Build history of the part. All positions in model axes, mm. Face numbers are marked on the shaded views. A direction names the side the tool comes from. Round coordinates to 2 decimals unless told otherwise and drop trailing zeros. Write each loop counter-clockwise with the first axis right and the second up, starting at its lowest first coordinate (ties: lowest second). Pieces come first, ordered by that corner, then holes. Notation, with made-up numbers: (63.25, 39.5) - (113.25, 39.5) arc R24 cw to (113.25, 78.5) - close; hole circle Ø9 at (-18.5, -12.75). An arc over 180 degrees is marked (long way). Write each question's results on one line, items separated by ' | '.
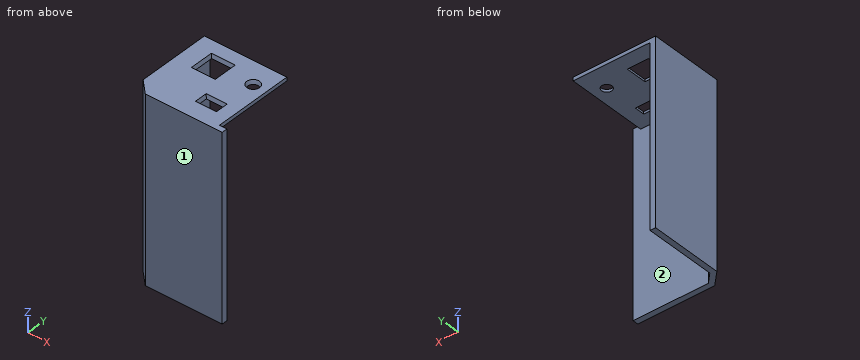
from build123d import *

# Parameters (mm, degrees)
BOSS_EXTRUDE1_DEPTH          = 100
BOSS_EXTRUDE2_DEPTH          = 2
CUT_EXTRUDE2_REACH           = 120.237
SKETCH4_R                    = 2.75
CUT_EXTRUDE3_REACH           = 120.237
SKETCH5_W                    = 9
SKETCH5_H                    = 4
CUT_EXTRUDE4_REACH           = 120.237
SKETCH6_W                    = 10
SKETCH6_H                    = 10
SKETCH7_R                    = 3.5
CUT_EXTRUDE6_DEPTH           = 2
CUT_EXTRUDE6_DRAFT           = -20
SKETCH7_W                    = 11.447026043
SKETCH7_H                    = 7
CUT_EXTRUDE6_PROFILE_2_DEPTH = 2
CUT_EXTRUDE6_PROFILE_2_DRAFT = -20
SKETCH7_W_2                  = 13
SKETCH7_H_2                  = 13
CUT_EXTRUDE6_PROFILE_3_DEPTH = 2
CUT_EXTRUDE6_PROFILE_3_DRAFT = -20


with BuildPart() as part:
    # Sketch2 → Boss-Extrude1 (new body)
    with BuildSketch(Plane.XY):
        Polygon((-7.071067812, 47.073759399), (-4.071067812, 47.073759399), (-4.071067812, 8.071067812), (1, 3), (42, 3), (42, 0), (0, 0), (-7.071067812, 7.071067812), align=None)
    extrude(amount=BOSS_EXTRUDE1_DEPTH)

    # Sketch3 → Boss-Extrude2 (add)
    with BuildSketch(Plane.XY.offset(100)):
        Polygon((-4.071067812, 47.073759399), (37.928932188, 47.073759399), (37.928932188, 3), (1, 3), (-4.071067812, 8.071067812), align=None)
    extrude(amount=-BOSS_EXTRUDE2_DEPTH)

    # Sketch4 → Cut-Extrude2 (cut, up to next)
    with BuildSketch(Plane.XY.offset(100), mode=Mode.PRIVATE) as cut_extrude2_sk1:
        with Locations((30.428932188, 34.073759399)):
            Circle(SKETCH4_R)
    cut_extrude2_tool1 = extrude(cut_extrude2_sk1.sketch, amount=-CUT_EXTRUDE2_REACH, mode=Mode.PRIVATE) & part.part
    add(cut_extrude2_tool1.solids().sort_by_distance((30.428932, 34.073759, 100))[0], mode=Mode.SUBTRACT)

    # Sketch5 → Cut-Extrude3 (cut, up to next)
    with BuildSketch(Plane.XY.offset(100), mode=Mode.PRIVATE) as cut_extrude3_sk1:
        with Locations((25.428932188, 13)):
            Rectangle(SKETCH5_W, SKETCH5_H)
    cut_extrude3_tool1 = extrude(cut_extrude3_sk1.sketch, amount=-CUT_EXTRUDE3_REACH, mode=Mode.PRIVATE) & part.part
    add(cut_extrude3_tool1.solids().sort_by_distance((25.428932, 13, 100))[0], mode=Mode.SUBTRACT)

    # Sketch6 → Cut-Extrude4 (cut, up to next)
    with BuildSketch(Plane.XY.offset(100), mode=Mode.PRIVATE) as cut_extrude4_sk1:
        with Locations((9.428932188, 33.144002223)):
            Rectangle(SKETCH6_W, SKETCH6_H)
    cut_extrude4_tool1 = extrude(cut_extrude4_sk1.sketch, amount=-CUT_EXTRUDE4_REACH, mode=Mode.PRIVATE) & part.part
    add(cut_extrude4_tool1.solids().sort_by_distance((9.428932, 33.144002, 100))[0], mode=Mode.SUBTRACT)


with BuildPart() as cut_extrude6_tool:
    # Sketch7 → Cut-Extrude6 (with draft: the straight prism first)
    with BuildSketch(Plane.XY.offset(100)):
        with Locations((30.428932188, 34.073759399)):
            Circle(SKETCH7_R)
    extrude(amount=-CUT_EXTRUDE6_DEPTH)
    # Cut-Extrude6: the draft: its side faces are tilted about the plane it starts from
    cut_extrude6_sides = [cut_extrude6_tool.faces().sort_by_distance(p)[0] for p in [
        (26.928932188, 34.073759399, 99),
    ]]
    draft(cut_extrude6_sides, Plane.XY.offset(100), CUT_EXTRUDE6_DRAFT)


with BuildPart() as part_1:
    add(part.part)

    # Cut-Extrude6: cut by cut_extrude6_tool
    add(cut_extrude6_tool.part, mode=Mode.SUBTRACT)


with BuildPart() as cut_extrude6_profile_2_tool:
    # Sketch7 → Cut-Extrude6 profile 2 (with draft: the straight prism first)
    with BuildSketch(Plane.XY.offset(100)):
        with Locations((25.15244521, 13)):
            Rectangle(SKETCH7_W, SKETCH7_H)
    extrude(amount=-CUT_EXTRUDE6_PROFILE_2_DEPTH)
    # Cut-Extrude6 profile 2: the draft: its side faces are tilted about the plane it starts from
    cut_extrude6_profile_2_sides = [cut_extrude6_profile_2_tool.faces().sort_by_distance(p)[0] for p in [
        (19.428932188, 13, 99),
        (25.15244521, 9.5, 99),
        (30.875958231, 13, 99),
        (25.15244521, 16.5, 99),
    ]]
    draft(cut_extrude6_profile_2_sides, Plane.XY.offset(100), CUT_EXTRUDE6_PROFILE_2_DRAFT)


with BuildPart() as part_2:
    add(part_1.part)

    # Cut-Extrude6 profile 2: cut by cut_extrude6_profile_2_tool
    add(cut_extrude6_profile_2_tool.part, mode=Mode.SUBTRACT)


with BuildPart() as cut_extrude6_profile_3_tool:
    # Sketch7 → Cut-Extrude6 profile 3 (with draft: the straight prism first)
    with BuildSketch(Plane.XY.offset(100)):
        with Locations((9.428932188, 33.144002223)):
            Rectangle(SKETCH7_W_2, SKETCH7_H_2)
    extrude(amount=-CUT_EXTRUDE6_PROFILE_3_DEPTH)
    # Cut-Extrude6 profile 3: the draft: its side faces are tilted about the plane it starts from
    cut_extrude6_profile_3_sides = [cut_extrude6_profile_3_tool.faces().sort_by_distance(p)[0] for p in [
        (2.928932188, 33.144002223, 99),
        (9.428932188, 26.644002223, 99),
        (15.928932188, 33.144002223, 99),
        (9.428932188, 39.644002223, 99),
    ]]
    draft(cut_extrude6_profile_3_sides, Plane.XY.offset(100), CUT_EXTRUDE6_PROFILE_3_DRAFT)


with BuildPart() as part_3:
    add(part_2.part)

    # Cut-Extrude6 profile 3: cut by cut_extrude6_profile_3_tool
    add(cut_extrude6_profile_3_tool.part, mode=Mode.SUBTRACT)


solid = part_3.part
(1) Drill centre lines: probe 1 along Z at (x, y) = (1, 36); probe 2 along X at (y, z) = (34, 77); probe 3 along Y at (x, z) = (20.5, 65). Where is each one in solid material? Low to high. Write a range as [from, to].
Worked answers:
probe 1: z = [98, 100] | probe 2: x = [-7.07, -4.07] | probe 3: y = [0, 3]
(2) Flat gauge pins, fed straight in: pin 1 Ø6 at (x, y) = (36, 21) entering from -Z; pin 2 Ø8 at (y, z) = (24.5, 51) entering from +X; pin 3 Ø2 at (y, z) = (21, 99) entering from +X. Where does each tip first touch, or does it go through?
Worked answers:
pin 1: stops at z = 98 | pin 2: stops at x = -4.07 | pin 3: stops at x = 37.93
(3) Slice it at D-D, the plane z = 46. Write the cut outline in (x, y).
Worked answers:
outline: (-7.07, 7.07) - (0, 0) - (42, 0) - (42, 3) - (1, 3) - (-4.07, 8.07) - (-4.07, 47.07) - (-7.07, 47.07) - close
(4) Slice it at B-B, the plane x = 25. Write the cut outline in (y, z), and give its area (3 significant figures).
Worked answers:
outline: (0, 0) - (3, 0) - (3, 98) - (10.23, 98) - (9.5, 100) - (0, 100) - close; (15.77, 98) - (47.07, 98) - (47.07, 100) - (16.5, 100) - close | area: 376 mm2
(5) Tool access for the marked faces 1 and 2: list every direction of +Z, -Z, +X, -X, +Y, -Y with a clear straight run to the whole face (end or side of a thin tool).
Worked answers:
face 1: +Z, -Z, +X, -X, -Y | face 2: -Z, +X, +Y
(6) Slice it at C-C, the plane y = 24.5. Write the cut outline in (x, z).
Worked answers:
outline: (-7.07, 0) - (-4.07, 0) - (-4.07, 98) - (37.93, 98) - (37.93, 100) - (-7.07, 100) - close
(7) Slice it at A-A, the plane y = 12.5. Write the cut outline in (x, z), and give its area (3 significant figures).
Worked answers:
outline: (-7.07, 0) - (-4.07, 0) - (-4.07, 98) - (20.16, 98) - (19.43, 100) - (-7.07, 100) - close; (30.15, 98) - (37.93, 98) - (37.93, 100) - (30.88, 100) - close | area: 363 mm2
